```python
from build123d import *
from build123d.topology import SkipClean

# Parameters (mm, degrees)
SKETCH_1_W          = 17
SKETCH_1_H          = 17
SKETCH_1_R          = 3.5
EXTRUDE_1_DEPTH     = 21
SKETCH_4_W          = 17
SKETCH_4_H          = 17
EXTRUDE_2_DEPTH     = 19
SKETCH_5_R          = 3
CUT_EXTRUDE_2_DEPTH = 21
SKETCH_7_W          = 17
SKETCH_7_H          = 2.364359037
EXTRUDE_3_DEPTH     = 15
CUT_EXTRUDE_5_DEPTH = 10
SKETCH_9_R          = 3
CUT_EXTRUDE_6_DEPTH = 10
EXTRUDE_START       = 5
SKETCH_12_R         = 8.5
EXTRUDE_4_DEPTH     = 5
EXTRUDE_START_2     = 1
SKETCH_13_R         = 8.5
EXTRUDE_5_DEPTH     = 1
SKETCH_15_R         = 5.512560125
SKETCH_15_R_2       = 2
EXTRUDE_6_DEPTH     = 5
EXTRUDE_START_3     = -7
SKETCH_16_R         = 4.074487064
SKETCH_16_R_2       = 2
EXTRUDE_7_DEPTH     = 7


with BuildPart() as part:
    # Эскиз1 → Бобышка-Вытянуть1 (new body)
    with BuildSketch(Plane.XY):
        Rectangle(SKETCH_1_W, SKETCH_1_H)
        with Locations(Location((0, 0, 0), (0, 0, 180))):
            Circle(SKETCH_1_R, mode=Mode.SUBTRACT)
    extrude(amount=EXTRUDE_1_DEPTH)

    # Эскиз4 → Бобышка-Вытянуть2 (add)
    with BuildSketch(Plane(origin=(0, 0, 0), x_dir=(-1, 0, 0), z_dir=(0, 0, -1))):
        Rectangle(SKETCH_4_W, SKETCH_4_H)
    extrude(amount=EXTRUDE_2_DEPTH)

    # Эскиз5 → Вырез-Вытянуть2 (cut)
    with BuildSketch(Plane(origin=(0, 0, -19), x_dir=(-1, 0, 0), z_dir=(0, 0, -1))):
        Circle(SKETCH_5_R)
    extrude(amount=-CUT_EXTRUDE_2_DEPTH, mode=Mode.SUBTRACT)

    # Эскиз7 → Бобышка-Вытянуть3 (add)
    with BuildSketch(Plane(origin=(0, 8.5, 0), x_dir=(1, 0, 0), z_dir=(0, 1, 0))):
        with Locations((0, -1.182179519)):
            Rectangle(SKETCH_7_W, SKETCH_7_H)
    extrude(amount=-EXTRUDE_3_DEPTH)

    # Эскиз10 → Вырез-Вытянуть5 (cut)
    with BuildSketch(Plane(origin=(0, 8.5, 0), x_dir=(1, 0, 0), z_dir=(0, 1, 0))):
        with BuildLine():
            Line((-7.050086148, -4), (-4.742367561, -4))
            ThreePointArc((-4.742367561, -4), (0, 0.742367561), (4.742367561, -4))
            Line((4.742367561, -4), (7.050086148, -4))
            ThreePointArc((7.050086148, -4), (0, 3.050086148), (-7.050086148, -4))
        make_face()
    extrude(amount=-CUT_EXTRUDE_5_DEPTH, mode=Mode.SUBTRACT)

    # Эскиз9 → Вырез-Вытянуть6 (cut)
    with BuildSketch(Plane(origin=(0, 8.5, 0), x_dir=(1, 0, 0), z_dir=(0, 1, 0))):
        with Locations(Location((0, -4, 0), (0, 0, 180))):
            Circle(SKETCH_9_R)
    extrude(amount=-CUT_EXTRUDE_6_DEPTH, mode=Mode.SUBTRACT)

    # Эскиз12 → Бобышка-Вытянуть4 (add)
    with SkipClean():  # the faces are left unmerged after this step: merging them gives an invalid solid
        with BuildSketch(Plane(origin=(0, 8.5, 0), x_dir=(1, 0, 0), z_dir=(0, 1, 0)).offset(EXTRUDE_START)):
            with Locations(Location((0, -4, 0), (0, 0, 180))):
                Circle(SKETCH_12_R)
            with BuildLine():
                ThreePointArc((-7.050086148, -4), (0, 3.050086148), (7.050086148, -4))
                ThreePointArc((7.050086148, -4), (0, -11.050086148), (-7.050086148, -4))
            make_face(mode=Mode.SUBTRACT)
        extrude(amount=-EXTRUDE_4_DEPTH)

    # Эскиз13 → Бобышка-Вытянуть5 (add)
    with SkipClean():  # the faces are left unmerged after this step: merging them gives an invalid solid
        with BuildSketch(Plane(origin=(0, 13.5, 0), x_dir=(1, 0, 0), z_dir=(0, 1, 0)).offset(EXTRUDE_START_2)):
            with Locations(Location((0, -4, 0), (0, 0, 180))):
                Circle(SKETCH_13_R)
        extrude(amount=-EXTRUDE_5_DEPTH)

    # Эскиз15 → Бобышка-Вытянуть6 (add)
    with SkipClean():  # the faces are left unmerged after this step: merging them gives an invalid solid
        with BuildSketch(Plane.XY.offset(21)):
            Circle(SKETCH_15_R)
            Circle(SKETCH_15_R_2, mode=Mode.SUBTRACT)
        extrude(amount=-EXTRUDE_6_DEPTH)

    # Эскиз16 → Бобышка-Вытянуть7 (add)
    with SkipClean():  # the faces are left unmerged after this step: merging them gives an invalid solid
        with BuildSketch(Plane(origin=(0, 0, -19), x_dir=(-1, 0, 0), z_dir=(0, 0, -1)).offset(EXTRUDE_START_3)):
            Circle(SKETCH_16_R)
            with Locations(Location((0, 0, 0), (0, 0, 180))):
                Circle(SKETCH_16_R_2, mode=Mode.SUBTRACT)
        extrude(amount=EXTRUDE_7_DEPTH)


solid = part.part
```
Build history of the part. All positions in model axes, mm. A direction names the side the tool comes from. Round coordinates to 2 decimals unless told otherwise and drop trailing zeros. Write each loop counter-clockwise with the first axis right and the second up, starting at its lowest first coordinate (ties: lowest second). Pieces come first, ordered by that corner, then holes. Notation, with made-up numbers: (12, 38.5) - (43, 38.5) arc R25 ccw to (43, 76.5) - close; hole circle Ø4 at (30.5, 42.5). An arc over 180 degrees is marked (long way). Write each question's results on one line, items separated by ' | '. Start each with the question number.
Item 1: Saw through at D-D (x = 4). Write the cut outline in (y, z), and give its area (3 significant figures).
Item 2: Saw through at C-C (y = 7.5). Write the cut outline in (x, z).
Item 3: Wall check: L1, parallel to Y at x = 0, z = 9.75; L2, parallel to Y at x = 0, z = -16.5; L3, parallel to X at y = 9.9, z = 4. Give the ranges that are in metal, low to high. Write a range as [from, to].
Item 4: Mould opens along Z. For faces 1 (the face through (0, 8.5, -10)), 2 (the face through (0.46, -3.47, 9.09)), 3 (the face through (0, 3, -0.3)), 4 (the face through (-2, 2, 21)) say: pulls with the +Z half, pulls with the -Z half, needs draft (parallel to the pull), parting line crosses it, or undercut.
Item 5: Saw through at B-B (z = -3.5). Write the cut outline in (x, y), and give its area (3 significant figures).
Item 6: Which spindle directions (+Z, -Z, +X, -X, +Y, -Y) get a long thin tool onto all of the face, cutting with end or side? Do faces 5 (the face through (0, -2, 2.364)), 6 (the face through (8.5, 0, 1)), 7 (the face through (0, 8.5, 16)), 8 (the face through (0, -2, 19)). Say none if no direction does.
Results are:
1) outline: (-8.5, -19) - (8.5, -19) - (8.5, -3.5) - (14.5, -3.5) - (14.5, 11.5) - (8.5, 11.5) - (8.5, 21) - (-8.5, 21) - close; hole (-1.5, -1.81) - (13.5, -1.81) - (13.5, 9.81) - (8.5, 9.81) - (8.5, 1.45) - (-1.5, 1.45) - close | area: 679 mm²
2) outline: (-8.5, -19) - (8.5, -19) - (8.5, 21) - (-8.5, 21) - close; hole (-7.05, 4) arc R7.05 ccw to (7.05, 4) - (4.74, 4) arc R4.74 cw to (-4.74, 4) - close; hole circle Ø6 at (0, 4)
3) L1: y = [-8.5, -3.5], [3.5, 8.5], [13.5, 14.5] | L2: y = [-8.5, -2], [2, 8.5] | L3: x = [-8.5, -7.05], [7.05, 8.5]
4) face 1: needs draft | face 2: undercut | face 3: undercut | face 4: pulls with the +Z half
5) outline: (-8.5, -8.5) - (8.5, -8.5) - (8.5, 8.5) - (4, 8.5) - (4, 14.5) - (-4, 14.5) - (-4, 8.5) - (-8.5, 8.5) - close; hole circle Ø6 at (0, 0) | area: 309 mm²
6) face 5: none | face 6: +Z, -Z, +X, +Y, -Y | face 7: +Z, +Y | face 8: +Z
